Geometry check sheet. Reference: the model listing, model coordinates, mm. A direction names the side the tool comes from. Coordinates: 2 decimals unless noted, no trailing zeros. Write each loop counter-clockwise with the first axis right and the second up, starting at its lowest first coordinate (ties: lowest second). Pieces come first, ordered by that corner, then holes. Notation, with made-up numbers: (30.5, 39.25) -> (73.5, 39.25) arc R24 cw to (73.5, 61.25) -> close; hole circle Ø9 at (-31.5, 81.5). An arc over 180 degrees is marked (long way). Answer in a Markdown table with one row per item. Add a question column.
Q1. Release check for a two-part mould opening along Z. For faces 1 (the face through (-3.007, 3.905, -0.867)), 2 (the face through (-2.34, 3.955, -5.158)), 3 (the face through (-3.5, 1, -2)) record: pulls with the +Z half, pulls with the -Z half, needs draft (parallel to the pull), parting line crosses it, or undercut.
Q2. Section check C-C, the plane x = -0.5. Record the boundary of the cut face in (y, z).
Q3. Thickness scan on line 1 (Y direction, x = 2.9, z = 0); line 2 (Y direction, x = 2.8, z = 0); line 3 (Z direction, x = 2.75, y = -2.75). Record the ranges inside material, lowest first.
Q4. Gauge pin test, flat ends, axial feed: P1, Ø1.5, axis at x = -1.5, y = 4, coming from the +Z side; P2, Ø3, axis at y = 0, z = 0, coming from the -X side. Record the tip position at first contact, or that the pin passes through.
Q5. Section check D-D, the plane x = 0.25. Record the boundary of the cut face in (y, z).
Q6. Tool access check on faces 4 (the face through (0, 2, 0)), 5 (the face through (2.993, 3.905, -0.867)), 6 (the face through (-3, 5, -1)). Record the directions out of +Z, -Z, +X, -X, +Y, -Y that give a thin tool (end or side, any length) a straight path to the whole face; none if there is none.
```python
from build123d import *

# Parameters (mm, degrees)
SKETCH_2_R = 2.5
FILLET_1_R = 0.3


with BuildPart() as part:
    # 草图1 → 旋转1 (revolve)
    with BuildSketch(Plane(origin=(0, 0, 0), x_dir=(1, 0, 0), z_dir=(0, 1, 0)), mode=Mode.PRIVATE) as revolve_1_sk:
        Polygon((-3.5, 2), (3.5, 2), (3.5, 4), (2.5, 4), (2.5, 4.75), (3, 4.75), (3, 6.5), (-3, 6.5), (-3, 4.75), (-2.5, 4.75), (-2.5, 4), (-3.5, 4), align=None)
    revolve(revolve_1_sk.sketch.rotate(Axis((0, 0, 0), (1, 0, 0)), 180), axis=Axis((0, 0, 0), (1, 0, 0)))

    # 草图2 → 切除-旋转1 (revolve, cut)
    with BuildSketch(Plane(origin=(0, 0, 0), x_dir=(1, 0, 0), z_dir=(0, 1, 0)), mode=Mode.PRIVATE) as cut_revolve_1_sk:
        with Locations((0, 8.04)):
            Circle(SKETCH_2_R)
    revolve(cut_revolve_1_sk.sketch.rotate(Axis((0, 0, 0), (-1, 0, 0)), 180), axis=Axis((0, 0, 0), (-1, 0, 0)), mode=Mode.SUBTRACT)

    # 圆角1
    fillet_1_edges = [part.edges().sort_by_distance(p)[0] for p in [
        (3, 0, -6.5),
        (-3, 0, -6.5),
    ]]
    fillet(fillet_1_edges, radius=FILLET_1_R)


solid = part.part
```
Calculated:
| question | item | result |
|---|---|---|
| 1 | face 1 | undercut |
| 1 | face 2 | parting line crosses it |
| 1 | face 3 | needs draft |
| 2 | outline | circle Ø11.18 at (0, 0); hole circle Ø4 at (0, 0) |
| 3 | line 1 | y = -6.42 to -4.75, -4 to -2, 2 to 4, 4.75 to 6.42 |
| 3 | line 2 | y = -6.48 to -4.75, -4 to -2, 2 to 4, 4.75 to 6.48 |
| 3 | line 3 | z = -5.88 to -3.87, -2.9 to 2.9, 3.87 to 5.88 |
| 4 | P1 | stops at z = 5.53 |
| 4 | P2 | passes through |
| 5 | outline | circle Ø11.11 at (0, 0); hole circle Ø4 at (0, 0) |
| 6 | face 4 | +X, -X |
| 6 | face 5 | +X |
| 6 | face 6 | -X |
